Drawing for the job (mm, zero at the part's lowest x, y, z). A direction names the side the tool comes from. Round coordinates to 2 decimals unless told otherwise and drop trailing zeros. Order: outer loops, then holes, each group sorted by start corner. A loop starts at its lowest first (then second) coordinate and runs counter-clockwise, first axis right, second up. Notation, with made-up numbers: (-3, 47) - (33, 47) arc R28 cw to (33, 86) - close; hole circle Ø11 at (29.5, 62.5). An arc over 180 degrees is marked (long way). Put each result on its own line as item: value. Start each with the question number.
Item 1: Probe probe 1 along Y at (x, z) = (15, 57); probe 2 along Z at (x, y) = (2, 38). List the from-to ranges inside material, lowest first.
Item 2: Which spindle directions (+Z, -Z, +X, -X, +Y, -Y) get a long thin tool onto all of the face, cutting with end or side? Do the marked faces 1 and 2. Say none if no direction does.
Item 3: Saw through at B-B on x = 21. List the corners of the cut face in (y, z).
Item 4: Saw through at A-A on z = 130. List the corners of the cut face in (x, y), plus the area to 3 significant figures.
Item 5: Saw through at C-C on y = 35.5. List the corners of the cut face in (x, z), plus the area to 3 significant figures.
Item 6: Pin check, flat tips, straight feed: pin 1 Ø11 at (y, z) = (21, 208) entering from +X; pin 2 Ø2 at (x, z) = (1.5, 15) entering from +Y; pin 3 Ø1.2 at (x, y) = (1.5, 28) entering from +Z. Stop position of each tip, or through.
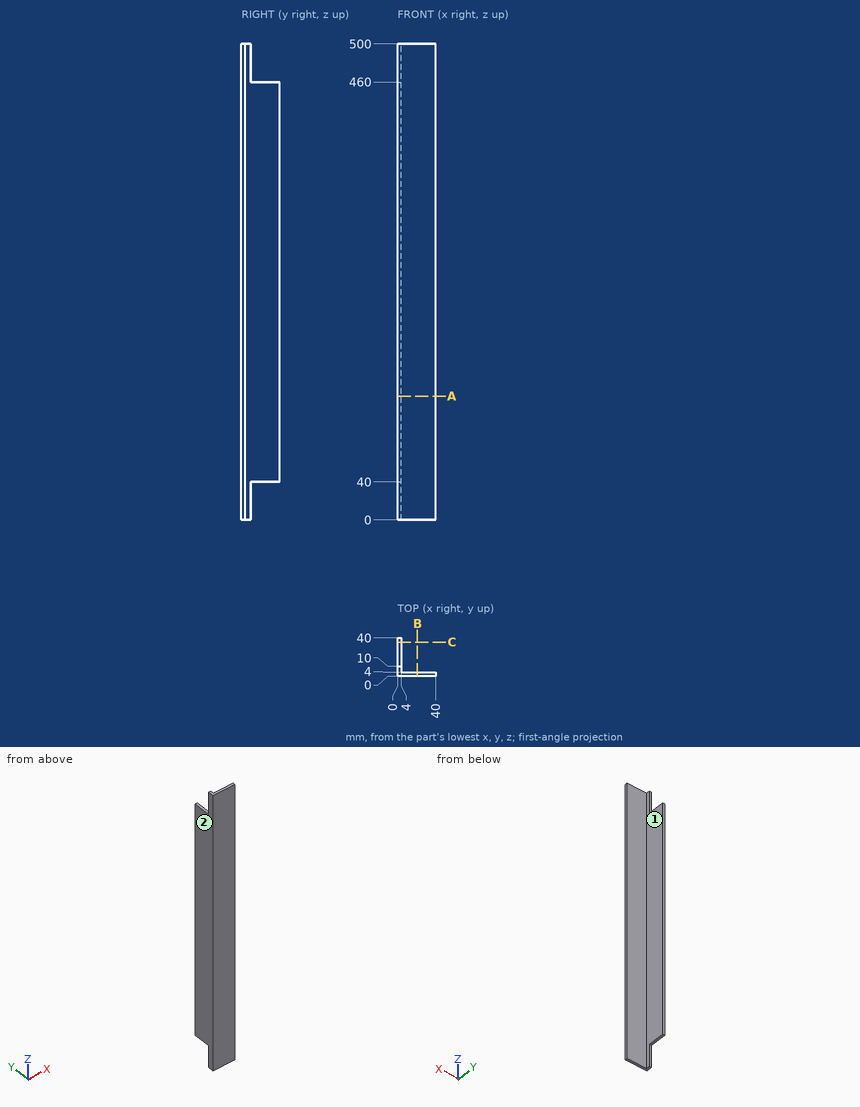
Results found:
1. probe 1: y = 0 to 4
1. probe 2: z = 40 to 460
2. face 1: +Z, -Z, +X, +Y
2. face 2: +Z, -Z, -X, +Y, -Y
3. outline: (0, 0) - (4, 0) - (4, 500) - (0, 500) - close
4. outline: (0, 0) - (40, 0) - (40, 4) - (4, 4) - (4, 40) - (0, 40) - close
4. area: 304 mm²
5. outline: (0, 40) - (4, 40) - (4, 460) - (0, 460) - close
5. area: 1,680 mm²
6. pin 1: stops at x = 4
6. pin 2: stops at y = 10
6. pin 3: stops at z = 460
